```python
from build123d import *

# Parameters (mm, degrees)
SKETCH1_W                = 65
SKETCH1_H                = 40
BOSS_EXTRUDE1_DEPTH      = 130
SHELL1_T                 = -4
FILLET1_R                = 5
CUT_EXTRUDE1_DEPTH       = 21
CUT_EXTRUDE1_DEPTH_BACK  = 21
SKETCH3_W                = 17.5
SKETCH3_H                = 50
CUT_EXTRUDE2_DEPTH       = 21
CUT_EXTRUDE2_DEPTH_BACK  = 21
SKETCH5_W                = 2
SKETCH5_H                = 50
BOSS_EXTRUDE2_DEPTH      = 3
SKETCH6_W                = 2
SKETCH6_H                = 30
BOSS_EXTRUDE3_DEPTH      = 3
SKETCH8_W                = 70
SKETCH8_H                = 66
BOSS_EXTRUDE4_DEPTH      = 20
SKETCH10_W               = 60
SKETCH10_H               = 12
CUT_EXTRUDE4_DEPTH       = 45
SKETCH23_W               = 2
SKETCH23_H               = 15
CUT_EXTRUDE10_DEPTH      = 10
SKETCH27_W               = 70
SKETCH27_H               = 33
CUT_EXTRUDE12_DEPTH      = 132.543487266
CUT_EXTRUDE12_DEPTH_BACK = 21
SKETCH31_R               = 2.7
CUT_EXTRUDE15_DEPTH      = 1
CUT_EXTRUDE15_DEPTH_BACK = 34
SKETCH33_R               = 4.5
CUT_EXTRUDE16_DEPTH      = 30
SKETCH34_R               = 1.7
CUT_EXTRUDE17_DEPTH      = 132.543487266
CUT_EXTRUDE17_DEPTH_BACK = 21
SKETCH35_R               = 4
CUT_EXTRUDE18_DEPTH      = 2
SKETCH41_W               = 6
SKETCH41_H               = 6
CUT_EXTRUDE21_DEPTH      = 3.5
CUT_EXTRUDE21_DEPTH_BACK = 68.5
SKETCH42_W               = 15
SKETCH42_H               = 17
BOSS_EXTRUDE10_DEPTH     = 2.5
SKETCH43_R               = 1.7
CUT_EXTRUDE22_DEPTH      = 3.5
CUT_EXTRUDE22_DEPTH_BACK = 10
SKETCH45_W               = 4.6
SKETCH45_H               = 4
BOSS_EXTRUDE11_DEPTH     = 3
CUT_EXTRUDE23_DEPTH      = 5
FILLET2_R                = 1
SKETCH49_R               = 1.7
CUT_EXTRUDE24_DEPTH      = 16.153953894
CUT_EXTRUDE24_DEPTH_BACK = 21
SKETCH50_W               = 15
SKETCH50_H               = 15
BOSS_EXTRUDE12_DEPTH     = 16
SKETCH52_R               = 4.2
CUT_EXTRUDE25_DEPTH      = 15
SKETCH53_R               = 2.7
CUT_EXTRUDE26_DEPTH      = 31.153953894
CUT_EXTRUDE26_DEPTH_BACK = 6


with BuildPart() as part:
    # Sketch1 → Boss-Extrude1 (new body)
    with BuildSketch(Plane(origin=(0, 0, 0), x_dir=(1, 0, 0), z_dir=(0, 1, 0))):
        Rectangle(SKETCH1_W, SKETCH1_H)
    extrude(amount=BOSS_EXTRUDE1_DEPTH)

    # Shell1
    shell1_openings = [part.faces().sort_by_distance(p)[0] for p in [
        (0, 130, 0),
        (0, 0, 0),
    ]]
    offset(amount=SHELL1_T, openings=shell1_openings, kind=Kind.INTERSECTION)

    # Fillet1
    fillet1_edges = [part.edges().sort_by_distance(p)[0] for p in [
        (32.5, 65, 20),
        (-32.5, 65, 20),
        (-32.5, 65, -20),
        (32.5, 65, -20),
    ]]
    fillet(fillet1_edges, radius=FILLET1_R)

    # Sketch2 → Cut-Extrude1 (cut, two sides)
    with BuildSketch(Plane.XY) as cut_extrude1_sk:
        Polygon((-5.5, 130), (-32.5, 85), (-32.5, 130), align=None)
    extrude(amount=CUT_EXTRUDE1_DEPTH, mode=Mode.SUBTRACT)
    extrude(cut_extrude1_sk.sketch, amount=-CUT_EXTRUDE1_DEPTH_BACK, mode=Mode.SUBTRACT)

    # Sketch3 → Cut-Extrude2 (cut, two sides)
    with BuildSketch(Plane.XY) as cut_extrude2_sk:
        with Locations((23.75, 105)):
            Rectangle(SKETCH3_W, SKETCH3_H)
    extrude(amount=CUT_EXTRUDE2_DEPTH, mode=Mode.SUBTRACT)
    extrude(cut_extrude2_sk.sketch, amount=-CUT_EXTRUDE2_DEPTH_BACK, mode=Mode.SUBTRACT)

    # Sketch5 → Boss-Extrude2 (add)
    with BuildSketch(Plane(origin=(15, 0, 0), x_dir=(0, 0, -1), z_dir=(1, 0, 0))):
        with Locations((-18, 105)):
            Rectangle(SKETCH5_W, SKETCH5_H)
    boss_extrude2 = extrude(amount=BOSS_EXTRUDE2_DEPTH)

    # Mirror1: Boss-Extrude2 across plane
    add(boss_extrude2.mirror(Plane.XY))

    # Sketch6 → Boss-Extrude3 (add)
    with BuildSketch(Plane(origin=(-61.397058824, 36.838235294, 0), x_dir=(0, 0, 1), z_dir=(-0.857492926, 0.514495755, 0))):
        with Locations((-18, 93.644353688)):
            Rectangle(SKETCH6_W, SKETCH6_H)
    boss_extrude3 = extrude(amount=BOSS_EXTRUDE3_DEPTH)

    # Mirror2: Boss-Extrude3 across plane
    add(boss_extrude3.mirror(Plane.XY))

    # Sketch8 → Boss-Extrude4 (add)
    with BuildSketch(Plane(origin=(0, 0, 0), x_dir=(1, 0, 0), z_dir=(0, 1, 0))):
        Rectangle(SKETCH8_W, SKETCH8_H)
    extrude(amount=-BOSS_EXTRUDE4_DEPTH)

    # Sketch10 → Cut-Extrude4 (cut)
    with BuildSketch(Plane.ZY.offset(35)):
        with Locations((0, -10)):
            Rectangle(SKETCH10_W, SKETCH10_H)
    extrude(amount=-CUT_EXTRUDE4_DEPTH, mode=Mode.SUBTRACT)

    # Sketch23 → Cut-Extrude10 (cut)
    with BuildSketch(Plane(origin=(0, 80, 0), x_dir=(1, 0, 0), z_dir=(0, 1, 0))):
        with Locations((30.5, 0)):
            Rectangle(SKETCH23_W, SKETCH23_H)
    extrude(amount=-CUT_EXTRUDE10_DEPTH, mode=Mode.SUBTRACT)

    # Sketch27 → Cut-Extrude12 (cut, two sides)
    with BuildSketch(Plane(origin=(0, 0, 0), x_dir=(1, 0, 0), z_dir=(0, 1, 0))) as cut_extrude12_sk:
        with Locations((0, -16.5)):
            Rectangle(SKETCH27_W, SKETCH27_H)
    extrude(amount=CUT_EXTRUDE12_DEPTH, mode=Mode.SUBTRACT)
    extrude(cut_extrude12_sk.sketch, amount=-CUT_EXTRUDE12_DEPTH_BACK, mode=Mode.SUBTRACT)

    # Sketch31 → Cut-Extrude15 (cut, two sides)
    with BuildSketch(Plane.XY) as cut_extrude15_sk:
        with Locations((27, -11)):
            Circle(SKETCH31_R)
    extrude(amount=CUT_EXTRUDE15_DEPTH, mode=Mode.SUBTRACT)
    extrude(cut_extrude15_sk.sketch, amount=-CUT_EXTRUDE15_DEPTH_BACK, mode=Mode.SUBTRACT)

    # Sketch33 → Cut-Extrude16 (cut)
    with BuildSketch(Plane(origin=(0, 0, -33), x_dir=(-1, 0, 0), z_dir=(0, 0, -1))):
        with Locations((-27, -11)):
            Circle(SKETCH33_R)
    extrude(amount=-CUT_EXTRUDE16_DEPTH, mode=Mode.SUBTRACT)

    # Sketch34 → Cut-Extrude17 (cut, two sides)
    with BuildSketch(Plane(origin=(0, 0, 0), x_dir=(1, 0, 0), z_dir=(0, 1, 0))) as cut_extrude17_sk:
        with Locations((0, 27)):
            Circle(SKETCH34_R)
    extrude(amount=CUT_EXTRUDE17_DEPTH, mode=Mode.SUBTRACT)
    extrude(cut_extrude17_sk.sketch, amount=-CUT_EXTRUDE17_DEPTH_BACK, mode=Mode.SUBTRACT)

    # Sketch35 → Cut-Extrude18 (cut)
    with BuildSketch(Plane(origin=(0, -20, 0), x_dir=(-1, 0, 0), z_dir=(0, -1, 0))):
        with Locations((0, 27)):
            Circle(SKETCH35_R)
    extrude(amount=-CUT_EXTRUDE18_DEPTH, mode=Mode.SUBTRACT)

    # Sketch41 → Cut-Extrude21 (cut, two sides)
    with BuildSketch(Plane(origin=(32.5, 0, 0), x_dir=(0, 0, -1), z_dir=(1, 0, 0))) as cut_extrude21_sk:
        with Locations((3, 20)):
            Rectangle(SKETCH41_W, SKETCH41_H)
    extrude(amount=CUT_EXTRUDE21_DEPTH, mode=Mode.SUBTRACT)
    extrude(cut_extrude21_sk.sketch, amount=-CUT_EXTRUDE21_DEPTH_BACK, mode=Mode.SUBTRACT)

    # Sketch42 → Boss-Extrude10 (add)
    with BuildSketch(Plane(origin=(32.5, 0, 0), x_dir=(0, 0, -1), z_dir=(1, 0, 0))):
        with Locations((7.5, 8.5)):
            Rectangle(SKETCH42_W, SKETCH42_H)
    extrude(amount=BOSS_EXTRUDE10_DEPTH)

    # Sketch43 → Cut-Extrude22 (cut, two sides)
    with BuildSketch(Plane(origin=(32.5, 0, 0), x_dir=(0, 0, -1), z_dir=(1, 0, 0))) as cut_extrude22_sk:
        with Locations((4, 76)):
            Circle(SKETCH43_R)
    extrude(amount=CUT_EXTRUDE22_DEPTH, mode=Mode.SUBTRACT)
    extrude(cut_extrude22_sk.sketch, amount=-CUT_EXTRUDE22_DEPTH_BACK, mode=Mode.SUBTRACT)

    # Sketch45 → Boss-Extrude11 (add)
    with BuildSketch(Plane(origin=(0, 0, -33), x_dir=(-1, 0, 0), z_dir=(0, 0, -1))):
        with Locations((27.1, -18)):
            Rectangle(SKETCH45_W, SKETCH45_H)
    extrude(amount=BOSS_EXTRUDE11_DEPTH)

    # Sketch46 → Cut-Extrude23 (cut, through all)
    with BuildSketch(Plane(origin=(0, -16, 0), x_dir=(1, 0, 0), z_dir=(0, 1, 0))):
        Polygon((-29.4, 33), (-24.8, 36), (-29.4, 36), align=None)
    extrude(amount=-CUT_EXTRUDE23_DEPTH, mode=Mode.SUBTRACT)

    # Fillet2
    fillet2_edges = [part.edges().sort_by_distance(p)[0] for p in [
        (-24.8, -18, -36),
    ]]
    fillet(fillet2_edges, radius=FILLET2_R)

    # Sketch49 → Cut-Extrude24 (cut, two sides)
    with BuildSketch(Plane(origin=(0, 0, -20), x_dir=(-1, 0, 0), z_dir=(0, 0, -1))) as cut_extrude24_sk:
        with Locations((6.357492926, 118.852591966)):
            Circle(SKETCH49_R)
    extrude(amount=CUT_EXTRUDE24_DEPTH, mode=Mode.SUBTRACT)
    extrude(cut_extrude24_sk.sketch, amount=-CUT_EXTRUDE24_DEPTH_BACK, mode=Mode.SUBTRACT)

    # Sketch50 → Boss-Extrude12 (add)
    with BuildSketch(Plane.XY.offset(-16)):
        with Locations((-21, 7.5)):
            Rectangle(SKETCH50_W, SKETCH50_H)
    extrude(amount=BOSS_EXTRUDE12_DEPTH)

    # Sketch52 → Cut-Extrude25 (cut)
    with BuildSketch(Plane(origin=(0, 0, -20), x_dir=(-1, 0, 0), z_dir=(0, 0, -1))):
        with Locations((22.5, 5)):
            Circle(SKETCH52_R)
    extrude(amount=-CUT_EXTRUDE25_DEPTH, mode=Mode.SUBTRACT)

    # Sketch53 → Cut-Extrude26 (cut, two sides)
    with BuildSketch(Plane(origin=(0, 0, -5), x_dir=(-1, 0, 0), z_dir=(0, 0, -1))) as cut_extrude26_sk:
        with Locations((22.5, 5)):
            Circle(SKETCH53_R)
    extrude(amount=CUT_EXTRUDE26_DEPTH, mode=Mode.SUBTRACT)
    extrude(cut_extrude26_sk.sketch, amount=-CUT_EXTRUDE26_DEPTH_BACK, mode=Mode.SUBTRACT)


solid = part.part
```
Work out the finished part from the listing and answer in its coordinate system (mm). A direction names the side the tool comes from. Round coordinates to 2 decimals unless told otherwise and drop trailing zeros. Write each loop counter-clockwise with the first axis right and the second up, starting at its lowest first coordinate (ties: lowest second). Pieces come first, ordered by that corner, then holes.
1) Consider probe 1 along Y at (x, z) = (-22, -12); probe 2 along Y at (x, z) = (-15, -27.5); probe 3 along X at (y, z) = (54.5, -4.5). Determine where each line is inside the solid, lowest interval first.
2) A cutting plane is placed at C-C on y = 76. Determine the outline of the cut face in (x, z).
3) Which of the six approach directions +Z, -Z, +X, -X, +Y, -Y give full straight-line access (tool end or side, diameter ignored) to faces 5 (the face through (29, 74.5, -4.8)), 6 (the face through (-15, 118, -17)), 7 (the face through (32.5, 48, -7))?
4) A cutting plane is placed at B-B on y = -11. Determine the outline of the cut face in (x, z), and give its area (3 significant figures).
5) Determine the mould class of faces 1 (the face through (24.3, -10.9, -1.5)), 2 (the face through (27, -14, -3)), 3 (the face through (7, 0, -8)), 4 (the face through (31.5, 74, -4)) for opening direction Y: pulls with the +Y half, pulls with the -Y half, needs draft (parallel to the pull), parting line crosses it, or undercut.
6) A cutting plane is placed at D-D on x = 0. Determine the outline of the cut face in (y, z).
7) A cutting plane is placed at A-A on z = -27. Determine the outline of the cut face in (x, y), and give its area (3 significant figures).
8) Flat-ended cylindrical pins translate along their axes: P1, Ø5.5, axis at x = -12, y = 119.5, coming from the -Z side; P2, Ø3.5, axis at y = -9.5, z = -16.5, coming from the -X side; P3, Ø0.9, axis at x = 16.5, y = 114, coming from the +Z side; P4, Ø3, axis at x = 27, y = -11, coming from the +Z side. Find the tip coordinate at first contact, or state that the pin passes through.
Entries:
1. probe 1: y = -20 to -16, -4 to 0.83, 9.17 to 15
1. probe 2: y = -20 to -16, -4 to 0
1. probe 3: x = -32.5 to -28.5, 28.5 to 32.5
2. outline: (-32.5, -15) arc R5 ccw to (-27.5, -20) - (27.5, -20) arc R5 ccw to (32.5, -15) - (32.5, -5.7) - (31.5, -5.7) - (31.5, -7.5) - (29.5, -7.5) - (29.5, -5.7) - (28.5, -5.7) - (28.5, -16) - (-28.5, -16) - (-28.5, 0) - (-32.5, 0) - close; (28.5, -2.3) - (29.5, -2.3) - (29.5, 0) - (28.5, 0) - close; (31.5, -2.3) - (32.5, -2.3) - (32.5, 0) - (31.5, 0) - close
3. face 5: +X
3. face 6: +Z, -X, +Y
3. face 7: +Z, -Z, +X, +Y
4. outline: (-35, -33) - (22.5, -33) - (22.5, -3) - (24.3, -3) - (24.3, 0) - (10, 0) - (10, -30) - (-35, -30) - close; (29.7, -3) - (31.5, -3) - (31.5, -33) - (35, -33) - (35, 0) - (29.7, 0) - close
4. area: 674 mm2
5. face 1: undercut
5. face 2: undercut
5. face 3: pulls with the +Y half
5. face 4: needs draft
6. outline: (-20, -33) - (0, -33) - (0, -28.7) - (-4, -28.7) - (-4, -30) - (-16, -30) - (-16, -28.7) - (-18, -28.7) - (-18, -31) - (-20, -31) - close; (-20, -23) - (-18, -23) - (-18, -25.3) - (-16, -25.3) - (-16, 0) - (-20, 0) - close; (-4, -25.3) - (0, -25.3) - (0, -20) - (130, -20) - (130, -16) - (0, -16) - (0, 0) - (-4, 0) - close
7. outline: (-35, -20) - (-4, -20) - (-4, -18) - (-1.7, -18) - (-1.7, -16) - (-35, -16) - close; (-35, -4) - (-1.7, -4) - (-1.7, 0) - (-35, 0) - close; (1.7, -18) - (4, -18) - (4, -20) - (35, -20) - (35, 0) - (1.7, 0) - (1.7, -4) - (10, -4) - (10, -16) - (1.7, -16) - close; hole circle Ø9 at (27, -11)
7. area: 760 mm2
8. P1: stops at z = -20
8. P2: stops at x = 10
8. P3: stops at z = -17
8. P4: passes through
